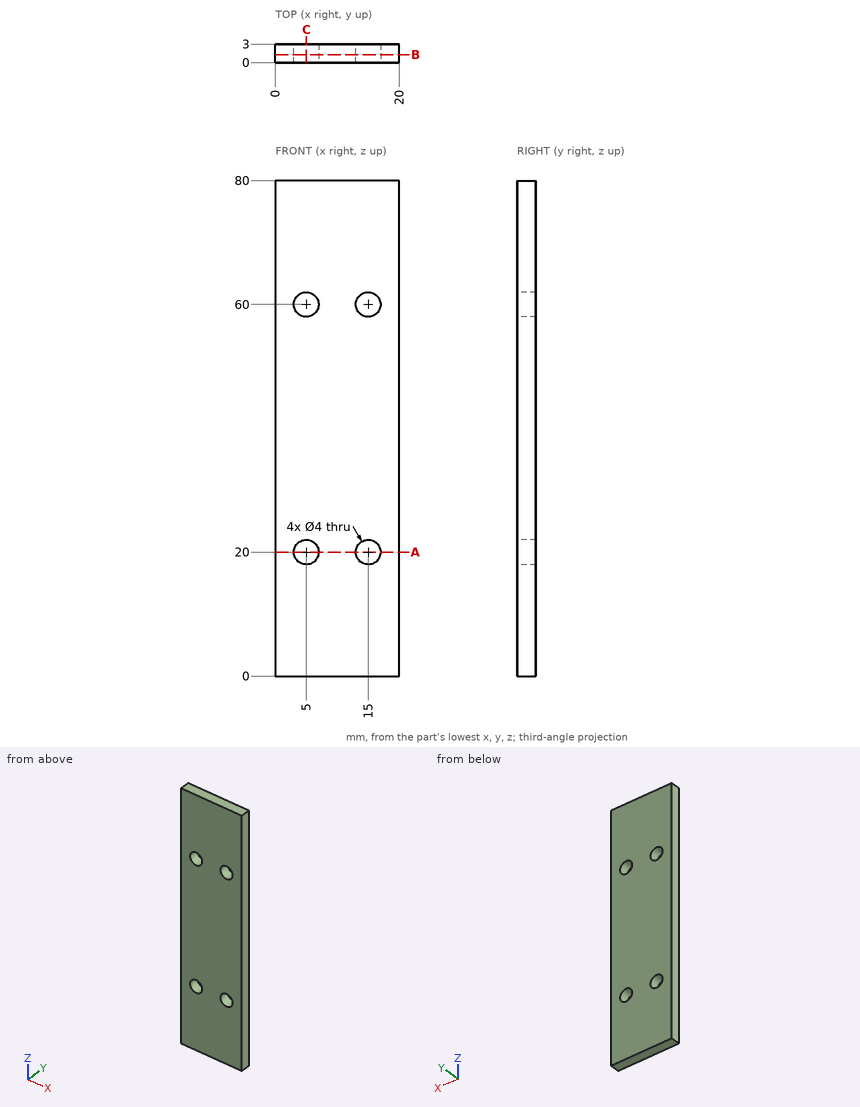
Job drawing, mm, ordinate dimensions from the low corner. One solid piece. Coordinates: 2 decimals unless noted, no trailing zeros. Order: outer loops, then holes, each group sorted by start corner. A loop starts at its lowest first (then second) coordinate and runs counter-clockwise, first axis right, second up. Notation, with made-up numbers: (34.5, 19.25) - (76.5, 19.25) arc R9 cw to (76.5, 31.25) - close; hole circle Ø7 at (34, 45.5). An arc over 180 degrees is marked (long way). Return JSON: item names as keys, results as strings. Group by question number.
1) Saw through at C-C, the plane x = 5. Write the cut outline in (y, z), plus the area to 3 significant figures.
2) Saw through at B-B, the plane y = 1.3. Write the cut outline in (x, z), plus the area to 3 significant figures.
3) Probe line 1 (Z direction, x = 5, y = 0.8); line 2 (X direction, y = 1.3, z = 19); line 3 (Z direction, x = 16.25, y = 0.8). List the from-to ranges inside material, lowest first. Write a range as from..to.
4) Flat gauge pin, fed straight in: P1, Ø1.5, axis at x = 15, z = 24, coming from the -Y side. Where does the tip first touch, or does it go through?
5) Saw through at A-A, the plane z = 20. Write the cut outline in (x, y), plus the area to 3 significant figures.
Values found:
{
 "1": {"outline": "(0, 0) - (3, 0) - (3, 18) - (0, 18) - close; (0, 22) - (3, 22) - (3, 58) - (0, 58) - close; (0, 62) - (3, 62) - (3, 80) - (0, 80) - close", "area": "216 mm²"},
 "2": {"outline": "(0, 0) - (20, 0) - (20, 80) - (0, 80) - close; hole circle Ø4 at (5, 20); hole circle Ø4 at (5, 60); hole circle Ø4 at (15, 20); hole circle Ø4 at (15, 60)", "area": "1,550 mm²"},
 "3": {"line 1": "z = 0..18, 22..58, 62..80", "line 2": "x = 0..3.27, 6.73..13.27, 16.73..20", "line 3": "z = 0..18.44, 21.56..58.44, 61.56..80"},
 "4": {"P1": "stops at y = 0"},
 "5": {"outline": "(0, 0) - (3, 0) - (3, 3) - (0, 3) - close; (7, 0) - (13, 0) - (13, 3) - (7, 3) - close; (17, 0) - (20, 0) - (20, 3) - (17, 3) - close", "area": "36.0 mm²"}
}
